Design review of the part built by this model. Coordinates are the model's own, in mm. A direction names the side the tool comes from. Coordinates: 2 decimals unless noted, no trailing zeros. Order: outer loops, then holes, each group sorted by start corner. A loop starts at its lowest first (then second) coordinate and runs counter-clockwise, first axis right, second up. Notation, with made-up numbers: (0, 14.5) -> (50, 14.5) arc R8 cw to (50, 22.5) -> close; hole circle Ø2 at (9.25, 47). An arc over 180 degrees is marked (long way). Write item = value, one per line.
```python
from build123d import *

# Parameters (mm, degrees)
BOSS_EXTRUDE1_DEPTH = 22.5
SKETCH2_R           = 5
BOSS_EXTRUDE2_DEPTH = 16.5
SKETCH3_W           = 13
SKETCH3_H           = 52.478254128
CUT_EXTRUDE1_DEPTH  = 76.539724649
SKETCH4_R           = 5
BOSS_EXTRUDE3_DEPTH = 6
SKETCH5_R           = 4
CUT_EXTRUDE2_DEPTH  = 100.582303751


with BuildPart() as part:
    # Sketch1 → Boss-Extrude1 (new, symmetric)
    with BuildSketch(Plane(origin=(0, 0, 0), x_dir=(0, 0, -1), z_dir=(1, 0, 0))):
        Polygon((0, 60), (0, 0), (-32, 0), (-32, 12), (-25, 12), (-25, 34.019237886), (-10, 60), align=None)
    extrude(amount=BOSS_EXTRUDE1_DEPTH, both=True)

    # Sketch2 → Boss-Extrude2 (add, symmetric)
    with BuildSketch(Plane(origin=(0, 0, 0), x_dir=(0, 0, -1), z_dir=(1, 0, 0))):
        with BuildLine():
            Line((0, 60), (30, 60))
            ThreePointArc((30, 60), (39.954230484, 50.95566494), (31.902581816, 40.182659096))
            Line((31.902581816, 40.182659096), (0, 34))
            Line((0, 34), (0, 60))
        make_face()
        with Locations((30, 50)):
            Circle(SKETCH2_R, mode=Mode.SUBTRACT)
    extrude(amount=BOSS_EXTRUDE2_DEPTH, both=True)

    # Sketch3 → Cut-Extrude1 (cut, through all)
    with BuildSketch(Plane(origin=(0, 60, 0), x_dir=(1, 0, 0), z_dir=(0, 1, 0))):
        with Locations((0, 26.239127064)):
            Rectangle(SKETCH3_W, SKETCH3_H)
    extrude(amount=-CUT_EXTRUDE1_DEPTH, mode=Mode.SUBTRACT)

    # Sketch4 → Boss-Extrude3 (add, symmetric)
    with BuildSketch(Plane(origin=(0, 0, 0), x_dir=(0, 0, -1), z_dir=(1, 0, 0))):
        with BuildLine():
            Line((-10, 60), (-39.932790381, 71.359051898))
            ThreePointArc((-39.932790381, 71.359051898), (-52.141016151, 67.009618943), (-49.803622697, 54.262268813))
            Line((-49.803622697, 54.262268813), (-25, 34.019237886))
            Line((-25, 34.019237886), (-10, 60))
        make_face()
        with Locations((-43.480762114, 62.009618943)):
            Circle(SKETCH4_R, mode=Mode.SUBTRACT)
    extrude(amount=BOSS_EXTRUDE3_DEPTH, both=True)

    # Sketch5 → Cut-Extrude2 (cut, through all)
    with BuildSketch(Plane.XY.offset(25)):
        with Locations((-13.5, 24)):
            Circle(SKETCH5_R)
        with Locations((13.5, 24)):
            Circle(SKETCH5_R)
    extrude(amount=-CUT_EXTRUDE2_DEPTH, mode=Mode.SUBTRACT)


solid = part.part
```
(1) We need section C-C (z = -16.5). Write out the cut boundary in (x, y).
Report:
outline = (-16.5, 37.2) -> (-6.5, 37.2) -> (-6.5, 60) -> (-16.5, 60) -> close; (6.5, 37.2) -> (16.5, 37.2) -> (16.5, 60) -> (6.5, 60) -> close
(2) The part is to be moulded in two halves that separate along Y. For faces 5 (the flat face through (0.1, 44.3, 37.6)), 6 (the flat face through (-22.5, 24, 12)), 7 (the flat face through (11.57, 37.135, -16.175)), 8 (the cylindrical face through (-11.43, 51.161, -39.932)), say which applies: released by +Y, released by -Y, zero draft, split by the parting line, or undercut.
Report:
face_5 = undercut
face_6 = zero draft
face_7 = released by -Y
face_8 = split by the parting line
(3) For faces 1 (the flat face through (14.366, 46.828, 17.605)), 2 (the flat face through (6.5, 50, -15)), 3 (the flat face through (0, 23, 25)), 4 (the flat face through (0, 60, 4)), list the 3-axis set-ups (+Z, -Z, +X, -X, +Y, -Y) from which the entire face can be reached by the end or side of a thin tool; tool diameter is ignored.
Report:
face_1 = +Z, +X, +Y
face_2 = -Z, +Y, -Y
face_3 = +Z, +X, -X
face_4 = -Z, +X, -X, +Y
(4) Insertion check: pin 1 (4 mm diameter, centred on x = 12.5, z = 30, fed in from -Y); pin 2 (3 mm diameter, centred on x = -14.5, y = 34, fed in from +Z); pin 3 (4 mm diameter, centred on x = -6.5, z = 34, fed in from +Y); pin 4 (12 mm diameter, centred on x = -7, y = 57.5, fed in from -Z). Each pin has a flat end and moves straight along its axis. Give the tip position at first contact, or say it passes through.
Report:
pin_1 = 0
pin_2 = 25
pin_3 = 69.84
pin_4 = -39.89
(5) We need section B-B (y = 24). Write out the cut boundary in (x, z), and give its area (3 significant figures).
Report:
outline = (-22.5, 0) -> (-17.5, 0) -> (-17.5, 25) -> (-22.5, 25) -> close; (-9.5, 0) -> (9.5, 0) -> (9.5, 25) -> (-9.5, 25) -> close; (17.5, 0) -> (22.5, 0) -> (22.5, 25) -> (17.5, 25) -> close
area = 725 mm²
(6) For L1, parallel to Y at x = 13.5, z = 8; L2, parallel to X at y = 56.5, z = -7; L3, parallel to Z at x = -15, y = 30.5, list the stretches that pass through material, from the lowest coordinate up.
Report:
L1 = 0 to 20, 28 to 60
L2 = -16.5 to -6.5, 6.5 to 16.5
L3 = 0 to 25
(7) We need section A-A (x = -13.5). Write out the cut boundary in (y, z).
Report:
outline = (0, 0) -> (20, 0) -> (20, 25) -> (12, 25) -> (12, 32) -> (0, 32) -> close; (28, 0) -> (34, 0) -> (40.18, -31.9) arc R10 ccw to (60, -30) -> (60, 10) -> (34.02, 25) -> (28, 25) -> close; hole circle Ø10 at (50, -30)
(8) We need section D-D (x = -19). Write out the cut boundary in (y, z).
Report:
outline = (0, 0) -> (60, 0) -> (60, 10) -> (34.02, 25) -> (12, 25) -> (12, 32) -> (0, 32) -> close
